Read the model definition and answer for the solid it produces. Units are mm, in the model's axes. A direction names the side the tool comes from. Give positions to 0.01 mm unless a question says otherwise; leave off trailing zeros. Write each loop counter-clockwise with the first axis right and the second up, starting at its lowest first coordinate (ties: lowest second). Pieces come first, ordered by that corner, then holes. Notation, with made-up numbers: (60.25, -7) -> (95.25, -7) arc R28 cw to (95.25, 17) -> close; hole circle Ø9 at (13.25, 82). An arc over 180 degrees is marked (long way). Put each result on its own line as item: value. Start each with the question number.
from build123d import *

# Parameters (mm, degrees)
SKETCH1_W           = 152.4
SKETCH1_H           = 45.72
BOSS_EXTRUDE1_DEPTH = 3.175
FILLET1_R           = 12.7
SKETCH2_R           = 0.999998
CUT_EXTRUDE1_DEPTH  = 4.175
SKETCH3_W           = 7.874
SKETCH3_H           = 3.175
CUT_EXTRUDE2_DEPTH  = 4.175
SKETCH4_W           = 10.35
SKETCH4_H           = 15
CUT_EXTRUDE3_DEPTH  = 4.175


with BuildPart() as part:
    # Sketch1 → Boss-Extrude1 (new body)
    with BuildSketch(Plane.XY):
        Rectangle(SKETCH1_W, SKETCH1_H)
    extrude(amount=BOSS_EXTRUDE1_DEPTH)

    # Fillet1
    fillet1_edges = [part.edges().sort_by_distance(p)[0] for p in [
        (-76.2, 22.86, 1.5875),
        (76.2, 22.86, 1.5875),
    ]]
    fillet(fillet1_edges, radius=FILLET1_R)

    # Sketch2 → Cut-Extrude1 (cut, through all)
    with BuildSketch(Plane.XY.offset(3.175)):
        with Locations((-57.15, -20.32)):
            Circle(SKETCH2_R)
        with Locations((-57.15, 20.32)):
            Circle(SKETCH2_R)
        with Locations((57.15, -20.32)):
            Circle(SKETCH2_R)
        with Locations((57.15, 20.32)):
            Circle(SKETCH2_R)
    extrude(amount=-CUT_EXTRUDE1_DEPTH, mode=Mode.SUBTRACT)

    # Sketch3 → Cut-Extrude2 (cut, through all)
    with BuildSketch(Plane.XY.offset(3.175)):
        with Locations((-44.45, -11.43)):
            Rectangle(SKETCH3_W, SKETCH3_H)
    extrude(amount=-CUT_EXTRUDE2_DEPTH, mode=Mode.SUBTRACT)

    # Sketch4 → Cut-Extrude3 (cut, through all)
    with BuildSketch(Plane.XY.offset(3.175)):
        with Locations((-44.45, 2.54)):
            Rectangle(SKETCH4_W, SKETCH4_H)
    extrude(amount=-CUT_EXTRUDE3_DEPTH, mode=Mode.SUBTRACT)


solid = part.part
1) A cutting plane is placed at A-A on y = 5.5. Give the vertices of the cut face in (x, z) (3 decimals).
2) A cutting plane is placed at B-B on z = 2.5. State how many separate pieces and enclosed holes the cut face has, and give its area (3 significant figures).
3) For a pull along X with two mould halves and no side action, classify faces 1 (the face through (76.2, -7, 2)), 2 (the face through (-76.2, -7, 2)), 3 (the face through (-45, -13.018, 2)) as pulls with the +X half, pulls with the -X half, needs draft (parallel to the pull), parting line crosses it, or undercut.
4) For faces 4 (the face through (-45, -9.842, 2)), 5 (the face through (-1, -22.86, 2)), determine the directions among +Z, -Z, +X, -X, +Y, -Y from which every point of the face is accessible in a straight line to the end or side of a thin tool.
5) Straight lines are drawn through the part: line 1 (Y direction, x = 57.15, z = 1.65); line 2 (X direction, y = 2, z = 1.4) (3 decimals); line 3 (Y direction, x = 67, z = 1.3). For each, find the intervals that lie inside material, in ascending order. Write a range as [from, to].
Results found:
1. outline: (-76.2, 0) -> (-49.625, 0) -> (-49.625, 3.175) -> (-76.2, 3.175) -> close; (-39.275, 0) -> (76.2, 0) -> (76.2, 3.175) -> (-39.275, 3.175) -> close
2. separate pieces: 1
2. enclosed holes: 6
2. area: 6,710 mm²
3. face 1: pulls with the +X half
3. face 2: pulls with the -X half
3. face 3: undercut
4. face 4: +Z, -Z
4. face 5: +Z, -Z, +X, -X, -Y
5. line 1: y = [-22.86, -21.32], [-19.32, 19.32], [21.32, 22.86]
5. line 2: x = [-76.2, -49.625], [-39.275, 76.2]
5. line 3: y = [-22.86, 22.37]
